Part model, mm, in its own coordinate system. A direction names the side the tool comes from. Give positions to 0.01 mm unless a question says otherwise; leave off trailing zeros. Write each loop counter-clockwise with the first axis right and the second up, starting at its lowest first coordinate (ties: lowest second). Pieces come first, ordered by that corner, then holes. Notation, with made-up numbers: M -27.5,23 L 24.5,23 A29 ccw 24.5,44 Z; hole C -18.75,29.25 d10. An arc over 180 degrees is marked long. Answer as CSV lines item,"result". Start each with the question number.
Item 1: Band-saw the part on C-C, the plane x = -3.5. List the corners of the cut face in (y, z), then the cut area to 3 significant figures.
Item 2: Two-plate mould, pull along Z, no slides. Class faces 1 (the flat face through (-3.75, 4, 0)), 2 (the flat face through (0, 5, -0.85)), 3 (the flat face through (0, -1, 5)): +Z half, -Z half, draft (parallel to the pull), parting line (faces both ways), or undercut.
Item 3: Band-saw the part on A-A, the plane z = 0. List the corners of the cut face in (x, y) (3 decimals), then the cut area to 3 significant figures.
Item 4: Band-saw the part on D-D, the plane y = 4.5. List the corners of the cut face in (x, z), then the cut area to 3 significant figures.
Item 5: Wall check: L1, parallel to X at y = -2, z = 0 (3 decimals); L2, parallel to X at y = 6.5, z = -0.5; L3, parallel to X at y = -0.75, z = 1.75. Give the ranges that are in metal, low to high. Write a range as from..to.
Item 6: Band-saw the part on B-B, the plane x = 9.5. List the corners of the cut face in (y, z), then the cut area to 3 significant figures.
Item 7: 3-axis set-ups, long thin cutter, end or side, ignore diameter. For faces 4 (the flat face through (-1.75, 5, 0)), 5 (the flat face through (-0.1, 9.5, 2.85)), 6 (the flat face through (10, 0, 1)): which of +Z, -Z, +X, -X, +Y, -Y reach the whole face in a straight line?
Item 8: Pin check, flat tips, straight feed: pin 1 (0.5 mm diameter, centred on x = -1, y = 9.5, fed in from +Z); pin 2 (0.5 mm diameter, centred on x = -1, y = 9.5, fed in from -Z); pin 3 (3 mm diameter, centred on x = -0.5, y = 7, fed in from +Z); pin 4 (3.5 mm diameter, centred on x = 7.875, z = 0, fed in from -Y). Stop position of each tip, or through.
from build123d import *

# Parameters (mm, degrees)
SKETCH1_W           = 7.5
SKETCH1_H           = 5.7
SKETCH1_W_2         = 3.5
SKETCH1_H_2         = 1.7
BOSS_EXTRUDE1_DEPTH = 10
SKETCH2_W           = 24
SKETCH2_H           = 10
BOSS_EXTRUDE2_DEPTH = 3
FILLET1_R           = 20
SKETCH3_R           = 2
CUT_EXTRUDE1_DEPTH  = 3


with BuildPart() as part:
    # Sketch1 → Boss-Extrude1 (new body)
    with BuildSketch(Plane(origin=(0, 0, 0), x_dir=(1, 0, 0), z_dir=(0, 1, 0))):
        Rectangle(SKETCH1_W, SKETCH1_H)
        Rectangle(SKETCH1_W_2, SKETCH1_H_2, mode=Mode.SUBTRACT)
    extrude(amount=BOSS_EXTRUDE1_DEPTH)

    # Sketch2 → Boss-Extrude2 (add)
    with BuildSketch(Plane.XZ):
        Rectangle(SKETCH2_W, SKETCH2_H)
    extrude(amount=BOSS_EXTRUDE2_DEPTH)

    # Fillet1
    # the kernel refuses this fillet: 20 mm, written as the material it adds along each edge
    with BuildSketch(Plane(origin=(3.75, 0, 2.85), x_dir=(0, 0, 1), z_dir=(-1, 0, 0)), Plane(origin=(-3.75, 0, -2.85), x_dir=(0, 0, -1), z_dir=(1, 0, 0))) as fillet1_piece_1:
        with BuildLine():
            CenterArc((20, 9.020947844), FILLET1_R, 180, 26.810903424)
            Line((0, 9.020947844), (-0.4, 9.020947844))
            Line((-0.4, 9.020947844), (-0.4, 0))
            Line((-0.4, 0), (0, -0.4))
            ThreePointArc((0, -0.4), (1.075, -0.4), (1.793, -0.180418957))
            Line((1.793, -0.180418957), (2.15, 0))
        make_face()
    extrude(amount=7.5)

    # Sketch3 → Cut-Extrude1 (cut)
    with BuildSketch(Plane(origin=(0, 0, 0), x_dir=(1, 0, 0), z_dir=(0, 1, 0))):
        with Locations(Location((-7.875, 0, 0), (0, 0, 270))):
            Circle(SKETCH3_R)
        with Locations(Location((7.875, 0, 0), (0, 0, 270))):
            Circle(SKETCH3_R)
    extrude(amount=-CUT_EXTRUDE1_DEPTH, mode=Mode.SUBTRACT)


solid = part.part
Output:
1,outline,"M -3,-5 L 0,-5 A20 cw 9.02,-2.85 L 10,-2.85 L 10,2.85 L 9.02,2.85 A20 cw 0,5 L -3,5 Z"
1,area,"99.6 mm²"
2,face 1,"draft"
2,face 2,"undercut"
2,face 3,"+Z half"
3,outline,"M -12,-3 L -9.875,-3 L -9.875,0 L -12,0 Z; M -5.875,-3 L 5.875,-3 L 5.875,0 L 3.75,0 L 3.75,10 L 1.75,10 L 1.75,0 L -1.75,0 L -1.75,10 L -3.75,10 L -3.75,0 L -5.875,0 Z; M 9.875,-3 L 12,-3 L 12,0 L 9.875,0 Z"
3,area,"88.0 mm²"
4,outline,"M -3.75,-3.37 L 3.75,-3.37 L 3.75,3.37 L -3.75,3.37 Z; hole M -1.75,-0.85 L 1.75,-0.85 L 1.75,0.85 L -1.75,0.85 Z"
4,area,"44.6 mm²"
5,L1,"-12..-9.875, -5.875..5.875, 9.875..12"
5,L2,"-3.75..-1.75, 1.75..3.75"
5,L3,"-12..-8.84, -6.91..6.91, 8.84..12"
6,outline,"M -3,-5 L 0,-5 L 0,-1.17 L -3,-1.17 Z; M -3,1.17 L 0,1.17 L 0,5 L -3,5 Z"
6,area,"23.0 mm²"
7,face 4,"+Y"
7,face 5,"+Z, +X, -X, +Y"
7,face 6,"+Z, -Z, +X, +Y"
8,pin 1,"z = 2.85"
8,pin 2,"z = -2.85"
8,pin 3,"z = 3.16"
8,pin 4,"through"
